Build history of the part. All positions in model axes, mm. Face numbers are marked on the shaded views. A direction names the side the tool comes from. Round coordinates to 2 decimals unless told otherwise and drop trailing zeros. Order: outer loops, then holes, each group sorted by start corner. A loop starts at its lowest first (then second) coordinate and runs counter-clockwise, first axis right, second up. Notation, with made-up numbers: (17.5, -25) -> (38.5, -25) arc R23 cw to (38.5, -3) -> close; hole circle Ø1 at (28.25, 54.5). An arc over 180 degrees is marked (long way). Use a Markdown table: item, result. Add a question column.
Item 1: Slice it at B-B, the plane z = 1.5. Give the cut face in (x, y).
Item 2: Slice it at D-D, the plane y = 9. Give the cut face in (x, z), plus the area to 3 significant figures.
Item 3: Probe L1, parallel to Y at x = 39, z = 2.5; L2, parallel to X at y = 1.5, z = 5.5; L3, parallel to Y at x = 0, z = 5. List the from-to ranges inside material, lowest first.
Item 4: Two-plate mould, pull along Y, no slides. Class the marked faces 1, 2 and 3: released by +Y, released by -Y, zero draft, split by the parting line, or undercut.
Item 5: 3-axis set-ups, long thin cutter, end or side, ignore diameter. For the marked faces 4, 5 and 6: which of +Z, -Z, +X, -X, +Y, -Y reach the whole face in a straight line?
Item 6: Pin check, flat tips, straight feed: pin 1 (16 mm diameter, centred on x = 38, y = -6, fed in from +Z); pin 2 (2 mm diameter, centred on y = 8.5, z = -2, fed in from +X); pin 3 (2.5 mm diameter, centred on x = -0.5, y = 1.5, fed in from +Z); pin 4 (10 mm diameter, centred on x = -19.5, y = 12, fed in from +Z). Stop position of each tip, or through.
Item 7: Slice it at A-A, the plane x = -39. Give the cut face in (y, z), plus the area to 3 significant figures.
Item 8: Slice it at C-C, the plane z = 15.5. Give the cut face in (x, y), plus the area to 3 significant figures.
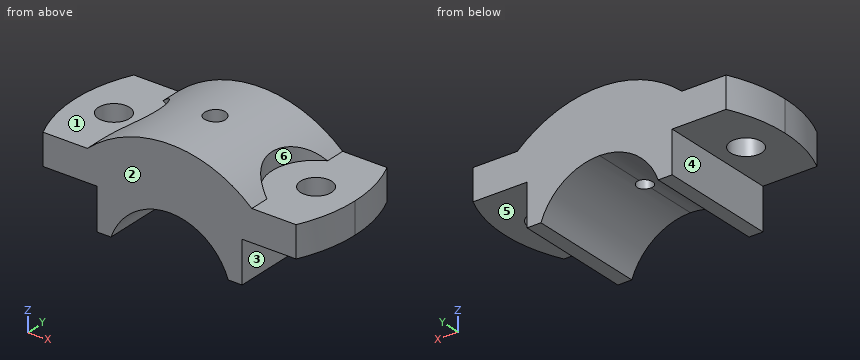
from build123d import *

# Parameters (mm, degrees)
F0_W           = 108
F0_H           = 12
F1_DEPTH       = 23
F3_DEPTH       = 23
F5_DEPTH       = 23
F6_R           = 6
F7_DEPTH       = 16.001
F7_DEPTH_BACK  = 25
F9_DEPTH       = 25
F10_R          = 4
F11_DEPTH      = 16
F12_R          = 3
F13_DEPTH      = 25
F13_DEPTH_BACK = 25
F15_DEPTH      = 25


with BuildPart() as f1:
    # F0 (on Front) → F1 (new body, symmetric)
    with BuildSketch(Plane.XZ):
        with Locations((0, 6)):
            Rectangle(F0_W, F0_H)
    extrude(amount=F1_DEPTH, both=True)

    # F2 (on Front) → F3 (join, symmetric)
    with BuildSketch(Plane.XZ):
        with BuildLine():
            ThreePointArc((-22.627416998, -16), (-13.8564064606, -4.4040820577), (0, 0))
            Line((0, 0), (-28, 0))
            Line((-28, 0), (-28, -16))
            Line((-28, -16), (-22.627416998, -16))
        make_face()
        with BuildLine():
            Line((28, -16), (28, 0))
            Line((28, 0), (0, 0))
            ThreePointArc((0, 0), (13.8564064606, -4.4040820577), (22.627416998, -16))
            Line((22.627416998, -16), (28, -16))
        make_face()
    extrude(amount=F3_DEPTH, both=True)

    # F4 (on Front) → F5 (join, symmetric)
    with BuildSketch(Plane.XZ):
        with BuildLine():
            ThreePointArc((31.7490157328, 12), (0, 24), (-31.7490157328, 12))
            Line((-31.7490157328, 12), (31.7490157328, 12))
        make_face()
    extrude(amount=F5_DEPTH, both=True)

    # F6 (on Top) → F7 (cut, two sides)
    with BuildSketch(Plane.XY) as f7_sk:
        with Locations((-39, 0)):
            Circle(F6_R)
        with Locations((39, 0)):
            Circle(F6_R)
    extrude(amount=-F7_DEPTH, mode=Mode.SUBTRACT)
    extrude(f7_sk.sketch, amount=F7_DEPTH_BACK, mode=Mode.SUBTRACT)

    # F8 (on face) → F9 (cut)
    with BuildSketch(Plane.XY.offset(12)):
        with BuildLine():
            ThreePointArc((31.7490157328, 15.3760601962), (22, 0), (31.7490157328, -15.3760601962))
            Line((31.7490157328, -15.3760601962), (31.7490157328, 15.3760601962))
        make_face()
        with BuildLine():
            Line((-31.7490157328, 15.3760601962), (-31.7490157328, -15.3760601962))
            ThreePointArc((-31.7490157328, -15.3760601962), (-22, 0), (-31.7490157328, 15.3760601962))
        make_face()
    extrude(amount=F9_DEPTH, mode=Mode.SUBTRACT)

    # F10 (on face) → F11 (cut)
    with BuildSketch(Plane.XY.offset(12)):
        Circle(F10_R)
    extrude(amount=F11_DEPTH, mode=Mode.SUBTRACT)

    # F12 (on face) → F13 (cut, two sides)
    with BuildSketch(Plane.XY.offset(12)) as f13_sk:
        Circle(F12_R)
    extrude(amount=-F13_DEPTH, mode=Mode.SUBTRACT)
    extrude(f13_sk.sketch, amount=F13_DEPTH_BACK, mode=Mode.SUBTRACT)

    # F14 (on face) → F15 (cut)
    with BuildSketch(Plane.XY.offset(12)):
        with BuildLine():
            ThreePointArc((-48.8569340012, -23), (-52.6985504358, -11.7840053448), (-54, 0))
            Line((-54, 0), (-54, -23))
            Line((-54, -23), (-48.8569340012, -23))
        make_face()
        with BuildLine():
            ThreePointArc((-54, 0), (-52.6985504358, 11.7840053448), (-48.8569340012, 23))
            Line((-48.8569340012, 23), (-54, 23))
            Line((-54, 23), (-54, 0))
        make_face()
        with BuildLine():
            ThreePointArc((54, 1.623e-07), (52.6985504535, -11.7840052656), (48.8569340012, -23))
            Line((48.8569340012, -23), (54, -23))
            Line((54, -23), (54, 1.623e-07))
        make_face()
        with BuildLine():
            ThreePointArc((48.8569340012, 23), (52.6985504181, 11.784005424), (54, 1.623e-07))
            Line((54, 1.623e-07), (54, 23))
            Line((54, 23), (48.8569340012, 23))
        make_face()
    extrude(amount=-F15_DEPTH, mode=Mode.SUBTRACT)


solid = f1.part
Check sheet entries:
| question | item | result |
|---|---|---|
| 1 | outline | (-48.86, -23) -> (48.86, -23) arc R54 ccw to (48.86, 23) -> (-48.86, 23) arc R54 ccw to start; hole circle Ø12 at (-39, 0); hole circle Ø6 at (0, 0); hole circle Ø12 at (39, 0) |
| 2 | outline | (-53.24, 0) -> (-28, 0) -> (-28, -16) -> (-22.63, -16) arc R24 cw to (22.63, -16) -> (28, -16) -> (28, 0) -> (53.24, 0) -> (53.24, 12) -> (24.58, 12) -> (24.58, 17.23) arc R48 ccw to (-24.58, 17.23) -> (-24.58, 12) -> (-53.24, 12) -> close |
| 2 | area | 2,130 mm2 |
| 3 | L1 | -23 to -6, 6 to 23 |
| 3 | L2 | -53.98 to -44.81, -33.19 to -2.6, 2.6 to 33.19, 44.81 to 53.98 |
| 3 | L3 | -23 to -3, 3 to 23 |
| 4 | face 1 | undercut |
| 4 | face 2 | released by -Y |
| 4 | face 3 | zero draft |
| 5 | face 4 | -Z, -X, +Y, -Y |
| 5 | face 5 | -Z, +X, +Y, -Y |
| 5 | face 6 | +Z, +X |
| 6 | pin 1 | z = 12 |
| 6 | pin 2 | x = 28 |
| 6 | pin 3 | through |
| 6 | pin 4 | z = 21.76 |
| 7 | outline | (-23, 0) -> (-6, 0) -> (-6, 12) -> (-23, 12) -> close; (6, 0) -> (23, 0) -> (23, 12) -> (6, 12) -> close |
| 7 | area | 408 mm2 |
| 8 | outline | (-27.27, -23) -> (27.27, -23) -> (27.27, -12.31) arc R17 cw to (27.27, 12.31) -> (27.27, 23) -> (-27.27, 23) -> (-27.27, 12.31) arc R17 cw to (-27.27, -12.31) -> close; hole circle Ø8 at (0, 0) |
| 8 | area | 2,280 mm2 |
